```python
from build123d import *

# Parameters (mm, degrees)
SKETCH_1_W          = 21
SKETCH_1_H          = 42.43
SKETCH_1_R          = 2.6
EXTRUDE_1_DEPTH     = 5
FILLET_1_R          = 10
SKETCH_3_W          = 30
SKETCH_3_H          = 7.5
CUT_EXTRUDE_2_DEPTH = 5


with BuildPart() as part:
    # 草图1 → 凸台-拉伸1 (new body)
    # profile 1 of 3: a face of its own
    with BuildSketch(Plane(origin=(0, 0, 0), x_dir=(1, 0, 0), z_dir=(0, 1, 0))):
        with Locations((-139.5, 0)):
            Rectangle(SKETCH_1_W, SKETCH_1_H)
        with Locations(Location((-132.3, 0, 0), (0, 0, 270))):
            Circle(SKETCH_1_R, mode=Mode.SUBTRACT)
    # profile 2 of 3: a face of its own
    with BuildSketch(Plane(origin=(0, 0, 0), x_dir=(1, 0, 0), z_dir=(0, 1, 0))):
        with BuildLine():
            Line((129, 21.215), (-129, 21.215))
            Line((-129, 21.215), (-129, -21.215))
            Line((-129, -21.215), (129, -21.215))
            Line((129, -21.215), (129, -2.4))
            ThreePointArc((129, -2.4), (127.4, 0), (129, 2.4))
            Line((129, 2.4), (129, 21.215))
        make_face()
    # profile 3 of 3: a face of its own
    with BuildSketch(Plane(origin=(0, 0, 0), x_dir=(1, 0, 0), z_dir=(0, 1, 0))):
        with BuildLine():
            Line((150, 21.215), (129, 21.215))
            Line((129, 21.215), (129, 2.4))
            ThreePointArc((129, 2.4), (131.44222051, 2.163330765), (132.6, 0))
            ThreePointArc((132.6, 0), (131.44222051, -2.163330765), (129, -2.4))
            Line((129, -2.4), (129, -21.215))
            Line((129, -21.215), (150, -21.215))
            Line((150, -21.215), (150, 21.215))
        make_face()
    extrude(amount=EXTRUDE_1_DEPTH)

    # 圆角1
    # the kernel refuses this fillet: 10 mm, written as the material it takes off along each edge
    with BuildSketch(Plane(origin=(150, 5, 42.865635095), x_dir=(-1, 0, 0), z_dir=(0, 0, -1)), Plane(origin=(-150, 5, -42.865635095), x_dir=(1, 0, 0), z_dir=(0, 0, 1))) as fillet_1_piece_1:
        with BuildLine():
            CenterArc((8.660254038, -10), FILLET_1_R, 90, 60)
            Line((0, -5), (-0.173205081, -4.9))
            ThreePointArc((-0.173205081, -4.9), (-0.2, -2.5), (-0.2, 0))
            Line((-0.2, 0), (0, 0.2))
            Line((0, 0.2), (8.660254038, 0.2))
            Line((8.660254038, 0.2), (8.660254038, 0))
        make_face()
    extrude(amount=85.731270189, mode=Mode.SUBTRACT)
    with BuildSketch(Plane(origin=(-171.650635095, 5, 21.215), x_dir=(0, 0, -1), z_dir=(1, 0, 0))) as fillet_1_piece_2:
        with BuildLine():
            CenterArc((8.660254038, -10), FILLET_1_R, 90, 60)
            Line((0, -5), (-0.173205081, -4.9))
            ThreePointArc((-0.173205081, -4.9), (-0.2, -2.5), (-0.2, 0))
            Line((-0.2, 0), (0, 0.2))
            Line((0, 0.2), (8.660254038, 0.2))
            Line((8.660254038, 0.2), (8.660254038, 0))
        make_face()
    extrude(amount=343.301270189, mode=Mode.SUBTRACT)
    with BuildSketch(Plane(origin=(-171.650635095, 5, -21.215), x_dir=(0, -1, 0), z_dir=(1, 0, 0))) as fillet_1_piece_3:
        with BuildLine():
            CenterArc((10, -8.660254038), FILLET_1_R, 120, 60)
            Line((0, -8.660254038), (-0.2, -8.660254038))
            Line((-0.2, -8.660254038), (-0.2, 0))
            Line((-0.2, 0), (0, 0.2))
            ThreePointArc((0, 0.2), (2.5, 0.2), (4.9, 0.173205081))
            Line((4.9, 0.173205081), (5, 0))
        make_face()
    extrude(amount=343.301270189, mode=Mode.SUBTRACT)

    # 草图3 → 切除-拉伸2 (cut)
    with BuildSketch(Plane(origin=(0, 5, 0), x_dir=(1, 0, 0), z_dir=(0, 1, 0))):
        with Locations((50, 3.75)):
            Rectangle(SKETCH_3_W, SKETCH_3_H)
        with Locations((50, -3.75)):
            Rectangle(SKETCH_3_W, SKETCH_3_H)
    extrude(amount=-CUT_EXTRUDE_2_DEPTH, mode=Mode.SUBTRACT)


solid = part.part
```
Input: part model. Units: mm. Frame: model coordinates. A direction names the side the tool comes from. Give positions to 0.01 mm unless a question says otherwise; leave off trailing zeros. Order: outer loops, then holes, each group sorted by start corner. A loop starts at its lowest first (then second) coordinate and runs counter-clockwise, first axis right, second up.
1. Mould query, pull axis X, two halves, no side actions, for faces 3 (the cylindrical face through (-146.276, 3.697, -0.297)), 4 (the cylindrical face through (-2.1, 3.62, -17.62)), 5 (the flat face through (50, 3, 7.5)), 6 (the cylindrical face through (-129.722, 2.465, -0.338)). Classes: released by +X, released by -X, zero draft, split by the parting line, or undercut.
Derived:
face 3: released by -X
face 4: zero draft
face 5: undercut
face 6: undercut
2. Section C-C on x = -132.3. Return the cut outline in (y, z) (3 decimals), and give its area (3 significant figures).
Derived:
outline: (0, -21.215) arc R10 ccw to (5, -12.555) - (5, -2.6) - (0, -2.6) - close; (0, 2.6) - (5, 2.6) - (5, 12.555) arc R10 ccw to (0, 21.215) - close
area: 161 mm2
3. Reachability of faces 1 (the flat face through (35, 3, 0)), 2 (the cylindrical face through (146.276, 3.697, 0.297)) from +Z, -Z, +X, -X, +Y, -Y: full face, straight path, thin tool, end or side. Return the list, or none.
Derived:
face 1: +Y, -Y
face 2: +Z, -Z, +X, +Y
4. Material intervals for L1, parallel to X at y = 1, z = 0; L2, parallel to X at y = 3.65, z = -1.5; L3, parallel to Z at x = -132.3, y = 1.85, sorted ascending.
Derived:
L1: x = -149.34 to -134.9, -129.7 to 35, 65 to 127.4, 132.6 to 149.34
L2: x = -146.36 to -134.42, -130.18 to 35, 65 to 127.88, 132.12 to 146.36
L3: z = -19.84 to -2.6, 2.6 to 19.84
5. Section B-B on y = 2.1. Return the cut outline in (x, z).
Derived:
outline: (-148.38, -19.6) - (148.38, -19.6) - (148.38, 19.6) - (-148.38, 19.6) - close; hole circle Ø5.2 at (-132.3, 0); hole (35, -7.5) - (65, -7.5) - (65, 7.5) - (35, 7.5) - close; hole circle Ø5.2 at (130, 0)
6. Pin query (flat end, axial travel): pin 1 (2.5 mm diameter, centred on y = 2.5, z = -1, fed in from +X); pin 2 (1.5 mm diameter, centred on x = 51, y = 2, fed in from -Z); pin 3 (1 mm diameter, centred on y = 3, z = 13, fed in from -X). Return the tip coordinate at first contact, or that it passes through.
Derived:
pin 1: stops at x = 149.15
pin 2: stops at z = -20.36
pin 3: stops at x = -147.95
7. Section A-A on x = 56. Return the cut outline in (y, z) (3 decimals).
Derived:
outline: (0, -21.215) arc R10 ccw to (5, -12.555) - (5, -7.5) - (0, -7.5) - close; (0, 7.5) - (5, 7.5) - (5, 12.555) arc R10 ccw to (0, 21.215) - close
